from build123d import *

# Parameters (mm, degrees)
SKETCH1_W           = 119.38
SKETCH1_H           = 122.682
BOSS_EXTRUDE1_DEPTH = 24.13
SKETCH2_W           = 15.24
SKETCH2_H           = 22.86
CUT_EXTRUDE1_DEPTH  = 139.549724374
CUT_EXTRUDE2_DEPTH  = 89.590033192
FILLET1_R           = 2.54


with BuildPart() as part:
    # Sketch1 → Boss-Extrude1 (new body)
    with BuildSketch(Plane.XY):
        Rectangle(SKETCH1_W, SKETCH1_H)
    extrude(amount=BOSS_EXTRUDE1_DEPTH)

    # Sketch2 → Cut-Extrude1 (cut, through all)
    with BuildSketch(Plane.XZ.offset(61.341)):
        with Locations((52.07, 12.7)):
            Rectangle(SKETCH2_W, SKETCH2_H)
        with Locations((-52.07, 12.7)):
            Rectangle(SKETCH2_W, SKETCH2_H)
    extrude(amount=-CUT_EXTRUDE1_DEPTH, mode=Mode.SUBTRACT)

    # Sketch3 → Cut-Extrude2 (cut, through all)
    with BuildSketch(Plane.XY.offset(1.27)):
        with BuildLine():
            Line((-59.69, 52.451), (-52.324, 52.451))
            ThreePointArc((-52.324, 52.451), (-49.911, 50.038), (-52.324, 47.625))
            Line((-52.324, 47.625), (-59.69, 47.625))
            ThreePointArc((-59.69, 47.625), (-62.103, 50.038), (-59.69, 52.451))
        make_face()
        with BuildLine():
            Line((-59.69, -47.625), (-52.324, -47.625))
            ThreePointArc((-52.324, -47.625), (-49.911, -50.038), (-52.324, -52.451))
            Line((-52.324, -52.451), (-59.69, -52.451))
            ThreePointArc((-59.69, -52.451), (-62.103, -50.038), (-59.69, -47.625))
        make_face()
        with BuildLine():
            Line((59.69, -52.451), (52.324, -52.451))
            ThreePointArc((52.324, -52.451), (49.911, -50.038), (52.324, -47.625))
            Line((52.324, -47.625), (59.69, -47.625))
            ThreePointArc((59.69, -47.625), (62.103, -50.038), (59.69, -52.451))
        make_face()
        with BuildLine():
            Line((59.69, 47.625), (52.324, 47.625))
            ThreePointArc((52.324, 47.625), (49.911, 50.038), (52.324, 52.451))
            Line((52.324, 52.451), (59.69, 52.451))
            ThreePointArc((59.69, 52.451), (62.103, 50.038), (59.69, 47.625))
        make_face()
    extrude(amount=-CUT_EXTRUDE2_DEPTH, mode=Mode.SUBTRACT)

    # Fillet1
    fillet1_edges = [part.edges().sort_by_distance(p)[0] for p in [
        (59.69, -61.341, 0.635),
        (-59.69, -61.341, 0.635),
        (-59.69, 61.341, 0.635),
        (59.69, 61.341, 0.635),
    ]]
    fillet(fillet1_edges, radius=FILLET1_R)


solid = part.part
Source: CAD feature listing. Evaluate the final solid. Frame: model axes, mm. A direction names the side the tool comes from. Round coordinates to 2 decimals unless told otherwise and drop trailing zeros. Loops run counter-clockwise (first coordinate to the right, second up) from the corner with the lowest first, then second, coordinate; pieces in that order, holes last. Notation, with made-up numbers: M 72.25,-16 L 128.25,-16 A16 cw 128.25,-7 Z; hole C 13.5,-19 d10. An arc over 180 degrees is marked long. Return JSON: item names as keys, results as strings. Group by question number.
1. Section query B-B on x = 46. Output: boundary loops of the cut face in (y, z), and give its area (3 significant figures).
2. Section query C-C on z = 10.5. Output: boundary loops of the cut face in (x, y).
3. Pin query (flat end, axial travel): pin 1 (4.5 mm diameter, centred on x = -55.5, y = 2, fed in from +Z); pin 2 (0.6 mm diameter, centred on x = 58, z = 0.5, fed in from +Y); pin 3 (5 mm diameter, centred on y = 6.5, z = 5, fed in from -X). Return the tip coordinate at first contact, or that it passes through.
4. Mould query, pull axis Z, two halves, no side actions, for faces 1 (the face through (-1, 1, 0)), 2 (the face through (52, -1, 1.27)), 3 (the face through (-44.45, -1, 13)). Classes: released by +Z, released by -Z, zero draft, split by the parting line, or undercut.
5. Material intervals for line 1 along Z through (x, y) = (55, -31.5); line 2 along X through (y, z) = (37.5, 3.75), sorted ascending. Write a range as from..to.
6. Section query A-A on y = -34. Output: boundary loops of the cut face in (x, z), and give its area (3 significant figures).
7. Reachability of faces 4 (the face through (-1, 61.341, 12)), 5 (the face through (44.45, -1, 13)), 6 (the face through (-52, -1, 1.27)) from +Z, -Z, +X, -X, +Y, -Y: full face, straight path, thin tool, end or side. Return the list, or none.
Checks:
{
 "1": {"outline": "M -61.34,0 L 61.34,0 L 61.34,1.27 L -61.34,1.27 Z", "area": "156 mm²"},
 "2": {"outline": "M -44.45,-61.34 L 44.45,-61.34 L 44.45,61.34 L -44.45,61.34 Z"},
 "3": {"pin 1": "stops at z = 1.27", "pin 2": "stops at y = 61.28", "pin 3": "stops at x = -44.45"},
 "4": {"face 1": "released by -Z", "face 2": "released by +Z", "face 3": "zero draft"},
 "5": {"line 1": "z = 0..1.27", "line 2": "x = -44.45..44.45"},
 "6": {"outline": "M -59.69,0 L 59.69,0 L 59.69,1.27 L 44.45,1.27 L 44.45,24.13 L -44.45,24.13 L -44.45,1.27 L -59.69,1.27 Z", "area": "2,180 mm²"},
 "7": {"face 4": "+Z, -Z, +X, -X, +Y", "face 5": "+Z, +X, +Y, -Y", "face 6": "+Z, -X, +Y, -Y"}
}
